Source: CAD feature listing. Evaluate the final solid. Frame: model axes, mm. A direction names the side the tool comes from. Give positions to 0.01 mm unless a question says otherwise; leave off trailing zeros. Order: outer loops, then holes, each group sorted by start corner. A loop starts at its lowest first (then second) coordinate and runs counter-clockwise, first axis right, second up. Notation, with made-up numbers: M 53,87.25 L 99,87.25 A31 cw 99,123.25 Z; hole C 71,-14.75 d6. An arc over 180 degrees is marked long. Answer as a JSON object with one key per item and string values. Group by question number.
1. Section query B-B (x = 11). Output: boundary loops of the cut face in (y, z).
2. Pin query (flat end, axial travel): P1, Ø4, axis at x = 29, z = -5, coming from the -Y side; P2, Ø8, axis at x = 11.5, z = 0, coming from the -Y side; P3, Ø2, axis at x = 44, z = -6.5, coming from the +Y side. Return the tip coordinate at first contact, or that it passes through.
3. Set-up query: faces 1 (the flat face through (3, 0, -8.5)), 2 (the cylindrical face through (15.48, -2.17, 9.76)), 3 (the flat face through (3.451, -7.327, -4.309)). Return all of +Z, -Z, +X, -X, +Y, -Y with unobstructed straight access to the full face (end or side cutting, diameter ignored); none if empty.
4. Section query A-A (x = 34.5). Output: boundary loops of the cut face in (y, z).
5. Section query D-D (x = 19.5). Output: boundary loops of the cut face in (y, z).
6. Pull-direction query (Y, two-part tool) for faces 4 (the cylindrical face through (36.818, -2.579, 1.978)), 5 (the flat face through (0, 4, -4)), 6 (the flat face through (3.451, 7.327, 4.309)); classes: +Y half, -Y half, draft (parallel to the pull), parting line (faces both ways), or undercut.
7. Material intervals for L1, parallel to Z at x = 3.25, y = 0; L2, parallel to Z at x = 37.5, y = 0, sorted ascending. Write a range as [from, to].
8. Section query C-C (x = 40). Output: boundary loops of the cut face in (y, z), plus the area to 3 significant figures.
from build123d import *

# Parameters (mm, degrees)
SCHNITT_LINEAR_AUSTRAGEN1_REACH = 54.364
SKIZZE2_R                       = 11


with BuildPart() as part:
    # Skizze1 → Rotation3 (revolve)
    with BuildSketch(Plane.XY):
        Polygon((1, 2), (50, 2), (50, 3.25), (24, 3.25), (24, 8.25), (45, 8.25), (45, 10), (42, 10), (39, 10.5), (20, 10.5), (17, 10), (14, 10), (14, 5.75), (13, 5.75), (13, 8), (7, 8), (7, 11), (0, 11), (0, 5.25), (8, 5.25), (8, 4.5), (1, 4.5), align=None)
    revolve(axis=Axis((92.390187717, 0, 0), (-1, 0, 0)))

    # Skizze2 → Schnitt-Linear austragen1 (cut, up to next)
    with BuildSketch(Plane.ZY, mode=Mode.PRIVATE) as schnitt_linear_austragen1_sk1:
        Circle(SKIZZE2_R)
        Polygon((-8.5, -4.907477288), (0, -9.814954576), (8.5, -4.907477288), (8.5, 4.907477288), (0, 9.814954576), (-8.5, 4.907477288), align=None, mode=Mode.SUBTRACT)
    schnitt_linear_austragen1_tool1 = extrude(schnitt_linear_austragen1_sk1.sketch, amount=-SCHNITT_LINEAR_AUSTRAGEN1_REACH, mode=Mode.PRIVATE) & part.part
    add(schnitt_linear_austragen1_tool1.solids().sort_by_distance((0, 0, -10.688873))[0], mode=Mode.SUBTRACT)


solid = part.part
Answer sheet:
{
 "1": {"outline": "C 0,0 d16; hole C 0,0 d4"},
 "2": {"P1": "y = -10.06", "P2": "y = -10", "P3": "y = 8.35"},
 "3": {"face 1": "-Z, -X, +Y, -Y", "face 2": "-X", "face 3": "-Z, -X, -Y"},
 "4": {"outline": "C 0,0 d21; C 0,0 d6.5; hole C 0,0 d16.5; hole C 0,0 d4"},
 "5": {"outline": "C 0,0 d20.83; hole C 0,0 d4"},
 "6": {"face 4": "undercut", "face 5": "draft", "face 6": "+Y half"},
 "7": {"L1": "[-8.5, -5.25], [-4.5, -2], [2, 4.5], [5.25, 8.5]", "L2": "[-10.5, -8.25], [-3.25, -2], [2, 3.25], [8.25, 10.5]"},
 "8": {"outline": "C 0,0 d20.67; C 0,0 d6.5; hole C 0,0 d16.5; hole C 0,0 d4", "area": "142 mm^2"}
}
